Autodesk Inventor part; units mm, degrees
ref_plane "YZ Plane" through (0, 0, 0) normal (1, 0, 0) x (0, 1, 0)
ref_plane "XZ Plane" through (0, 0, 0) normal (0, 1, 0) x (-1, 0, 0)
ref_plane "XY Plane" through (0, 0, 0) normal (0, 0, 1) x (1, 0, 0)
sketch "草圖1" plane through (0, 0, 0) normal (0, 1, 0) x (-1, 0, 0)
  circle A0 centre (0, 0) radius 20
  line L0 (0, -20) -> (30, -20)
  line L1 (30, -20) -> (30, 20)
  line L2 (30, 20) -> (0, 20)
  line L3 (0, 20) -> (0, -20)
  point P0 (0, 20)
  dimension "d0" = 40
  dimension "d1" = 30
extrude "擠出1" add sketch "草圖1" along normal blind 40
sketch "草圖2" plane through (0, 40, 0) normal (0, 1, 0) x (1, 0, 0)
  line L0 (-30, 20) -> (0, 20)
  arc A0 (0, -20) -> (0, 20) centre (0, 0) ccw
  line L1 (0, -20) -> (-30, -20)
  line L2 (-30, -20) -> (-30, 20)
  line L3 (0, 27.0691) -> (-10, 27.0691)
  line L4 (-10, 27.0691) -> (-10, -29.9758)
  line L5 (-10, -29.9758) -> (0, -29.9758)
  line L6 (0, -29.9758) -> (0, 27.0691)
  dimension "d4" = 20
  dimension "d5" = 10
extrude "擠出2" cut sketch "草圖2" against normal blind 10 contours L4 L3 L6 L0 | L0 L6 L1 L4 | L1 L6 L5 L4
sketch "草圖3" plane through (0, 40, 0) normal (0, 1, 0) x (1, 0, 0)
  line L0 (0, -20) -> (0, 20)
  arc A0 (0, -20) -> (0, 20) centre (0, 0) ccw
  line L1 (-10, 20) -> (-10, -20)
  line L2 (-10, -20) -> (-30, -20)
  line L3 (-30, -20) -> (-30, 20)
  line L4 (-30, 20) -> (-10, 20)
  line L5 (0, -34.6108) -> (30.5971, -34.6108)
  line L6 (30.5971, -34.6108) -> (30.5971, 28.6775)
  line L7 (30.5971, 28.6775) -> (0, 28.6775)
  line L8 (0, 28.6775) -> (0, -34.6108)
  line L9 (0, 20) -> (0, -20)
extrude "擠出3" cut sketch "草圖3" against normal blind 30 contours L0 A0 | A0 L8 L7 L6 L5
sketch "草圖4" plane through (0, 0, 0) normal (0, -1, 0) x (1, 0, 0)
  arc A0 (0, -20) -> (0, 20) centre (0, 0) ccw
hole "孔1" at (0, 0, 0) direction (0, 1, 0) diameter 20 end through all
properties part number "34" material "鋼、碳鋼"
CAD build for the part. Positions are in the model's coordinates, mm. A direction names the side the tool comes from. Coordinates: 2 decimals unless noted, no trailing zeros. Order: outer loops, then holes, each group sorted by start corner. A loop starts at its lowest first (then second) coordinate and runs counter-clockwise, first axis right, second up. Notation, with made-up numbers: M 2.25,3 L 41.25,3 A12 cw 41.25,15 Z; hole C 6,10 d10. An arc over 180 degrees is marked long. Answer as CSV lines item,"result".
1) Cut at A-A (z = -7.5). List the corners of the cut face in (x, y), then the cut area to 3 significant figures.
Verdict:
outline,"M -30,0 L -6.61,0 L -6.61,30 L -10,30 L -10,40 L -30,40 Z; M 6.61,0 L 18.54,0 L 18.54,10 L 6.61,10 Z"
area,"1,020 mm2"
2) Mould opens along X. For faces 1 (the flat face through (-20, 40, 0)), 2 (the cylindrical face through (20, 5, 0)), 3 (the cylindrical face through (-9.915, 11.877, 1.302)) say: released by +X, released by -X, zero draft, split by the parting line, or undercut.
Verdict:
face 1,"zero draft"
face 2,"released by +X"
face 3,"undercut"
3) Cut at C-C (y = 24.5). List the corners of the cut face in (x, z).
Verdict:
outline,"M -30,-20 L 0,-20 L 0,-10 A10 cw 0,10 L 0,20 L -30,20 Z"
4) Drill centre lines: L1, parallel to X at y = 9, z = 0; L2, parallel to Z at x = -0.5, y = 11; L3, parallel to X at y = 15, z = 0. Where is each one in solid material? Low to high. Write a range as from..to.
Verdict:
L1,"-30..-10, 10..20"
L2,"-20..-9.99, 9.99..20"
L3,"-30..-10"
5) Cut at D-D (x = 12). List the corners of the cut face in (y, z), then the cut area to 3 significant figures.
Verdict:
outline,"M 0,-16 L 10,-16 L 10,16 L 0,16 Z"
area,"320 mm2"
6) Cut at B-B (y = 3). List the corners of the cut face in (x, z), then the cut area to 3 significant figures.
Verdict:
outline,"M -30,-20 L 0,-20 A20 ccw 0,20 L -30,20 Z; hole C 0,0 d20"
area,"1,510 mm2"
7) Flat gauge pins, fed straight in: P1, Ø3, axis at y = 33, z = 1.5, coming from the +X side; P2, Ø23, axis at x = 0, z = 0, coming from the -Y side; P3, Ø8, axis at y = 21, z = -17.5, coming from the +X side; P4, Ø10, axis at x = 7, z = 2, coming from the +Y side. Where does each tip first touch, or does it go through?
Verdict:
P1,"x = -10"
P2,"y = 0"
P3,"x = 0"
P4,"y = 10"
8) 3-axis set-ups, long thin cutter, end or side, ignore diameter. For faces 4 (the flat face through (0, 20, -15)), 5 (the flat face through (-30, 20, 0)): which of +Z, -Z, +X, -X, +Y, -Y reach the whole face in a straight line?
Verdict:
face 4,"+Z, -Z, +X, +Y"
face 5,"+Z, -Z, -X, +Y, -Y"
